```python
from build123d import *

# Parameters (mm, degrees)
SKETCH_1_W          = 13
SKETCH_1_H          = 26
SKETCH_1_R          = 1.5
SKETCH_1_W_2        = 14
SKETCH_1_H_2        = 30
EXTRUDE_1_DEPTH     = 3
SKETCH_2_R          = 21
CUT_EXTRUDE_1_DEPTH = 3
FILLET_1_R          = 5


with BuildPart() as part:
    # 草图1 → 凸台-拉伸1 (new body)
    # profile 1 of 3: a face of its own
    with BuildSketch(Plane.XY):
        Rectangle(SKETCH_1_W, SKETCH_1_H)
        with Locations((-3.5, 3)):
            Circle(SKETCH_1_R, mode=Mode.SUBTRACT)
        with Locations((-3.5, -3)):
            Circle(SKETCH_1_R, mode=Mode.SUBTRACT)
        with Locations((3.5, -3)):
            Circle(SKETCH_1_R, mode=Mode.SUBTRACT)
        with Locations((3.5, 3)):
            Circle(SKETCH_1_R, mode=Mode.SUBTRACT)
    # profile 2 of 3: a face of its own
    with BuildSketch(Plane.XY):
        Polygon((22, 28.52), (22, -1.48), (36, -1.48), (6.5, -13), (6.5, 13), (-6.5, 13), align=None)
    # profile 3 of 3: a face of its own
    with BuildSketch(Plane.XY):
        with Locations((29, 13.52)):
            Rectangle(SKETCH_1_W_2, SKETCH_1_H_2)
        with Locations((25, 21.52)):
            Circle(SKETCH_1_R, mode=Mode.SUBTRACT)
        with Locations((25, 5.52)):
            Circle(SKETCH_1_R, mode=Mode.SUBTRACT)
        with Locations((33, 5.52)):
            Circle(SKETCH_1_R, mode=Mode.SUBTRACT)
        with Locations((33, 21.52)):
            Circle(SKETCH_1_R, mode=Mode.SUBTRACT)
    extrude(amount=EXTRUDE_1_DEPTH)

    # 草图2 → 切除-拉伸1 (cut)
    with BuildSketch(Plane.XY.offset(3)):
        with Locations((-3.5, 28.52)):
            Circle(SKETCH_2_R)
    extrude(amount=-CUT_EXTRUDE_1_DEPTH, mode=Mode.SUBTRACT)

    # 圆角1
    fillet_1_edges = [part.edges().sort_by_distance(p)[0] for p in [
        (-6.5, -13, 1.5),
        (22, 28.52, 1.5),
        (36, 28.52, 1.5),
        (36, -1.48, 1.5),
        (6.5, -13, 1.5),
        (17.346543443, 25.985907166, 1.5),
        (-6.5, 7.735390309, 1.5),
    ]]
    fillet(fillet_1_edges, radius=FILLET_1_R)


solid = part.part
```
Geometry check sheet. Reference: the model listing, model coordinates, mm. Round coordinates to 2 decimals unless told otherwise and drop trailing zeros. Loops run counter-clockwise (first coordinate to the right, second up) from the corner with the lowest first, then second, coordinate; pieces in that order, holes last. Notation, with made-up numbers: (51, 87.5) - (86, 87.5) arc R31 ccw to (86, 123.5) - close; hole circle Ø2 at (-13.75, 23). An arc over 180 degrees is marked (long way). Use a Markdown table: item, result.
Q1. Cross-section at C-C on z = 2.15. State how many separate pieces and enclosed holes the cut face has, plus the area to 3 significant figures.
Solutions:
| item | result |
|---|---|
| separate pieces | 1 |
| enclosed holes | 8 |
| area | 1,100 mm2 |
Q2. Cross-section at D-D on y = 14. Record the cut outline in (x, z), plus the area to 3 significant figures.
Solutions:
| item | result |
|---|---|
| outline | (11.67, 0) - (36, 0) - (36, 3) - (11.67, 3) - close |
| area | 73.0 mm2 |
Q3. Go/stop test with a flat-tipped pin: P1, Ø1, axis at x = 1.5, z = 2, coming from the +Y side. Record where the tip stops, or that it passes through.
Solutions:
| item | result |
|---|---|
| P1 | stops at y = 8.25 |
Q4. Material ranges on line 1 (Y direction, x = 3, z = 0.8); line 2 (Y direction, x = 2.5, z = 2); line 3 (X direction, y = 6.5, z = 0.2), recorded low to high.
Solutions:
| item | result |
|---|---|
| line 1 | y = -13 to -4.41, -1.59 to 1.59, 4.41 to 8.55 |
| line 2 | y = -13 to -4.12, -1.88 to 1.88, 4.12 to 8.4 |
| line 3 | x = -4.63 to 23.86, 26.14 to 31.86, 34.14 to 36 |
Q5. Cross-section at A-A on y = 5.52. Record the cut outline in (x, z), plus the area to 3 significant figures.
Solutions:
| item | result |
|---|---|
| outline | (-5.56, 0) - (23.5, 0) - (23.5, 3) - (-5.56, 3) - close; (26.5, 0) - (31.5, 0) - (31.5, 3) - (26.5, 3) - close; (34.5, 0) - (36, 0) - (36, 3) - (34.5, 3) - close |
| area | 107 mm2 |
Q6. Cross-section at B-B on x = -3.5. Record the cut outline in (y, z), plus the area to 3 significant figures.
Solutions:
| item | result |
|---|---|
| outline | (-12.58, 0) - (-4.5, 0) - (-4.5, 3) - (-12.58, 3) - close; (-1.5, 0) - (1.5, 0) - (1.5, 3) - (-1.5, 3) - close; (4.5, 0) - (7.18, 0) - (7.18, 3) - (4.5, 3) - close |
| area | 41.3 mm2 |
Q7. Draft check along X on faces 1 (the flat face through (2, -13, 1)), 2 (the cylindrical face through (6.5, -12.91, 1.52)), 3 (the cylindrical face through (31.5, 5.59, 1.48)), 4 (the flat face through (20.16, 27.52, 1.48)). Enter one of: released by +X, released by -X, zero draft, split by the parting line, or undercut.
Solutions:
| item | result |
|---|---|
| face 1 | zero draft |
| face 2 | released by +X |
| face 3 | undercut |
| face 4 | released by -X |
